Here's how the part is built. I have some questions about the finished solid (model axes, mm). Face numbers are marked on the shaded views. A direction names the side the tool comes from. Round coordinates to 2 decimals unless told otherwise and drop trailing zeros. Order: outer loops, then holes, each group sorted by start corner. A loop starts at its lowest first (then second) coordinate and runs counter-clockwise, first axis right, second up. Notation, with made-up numbers: (-21, -10) -> (14, -10) arc R14 ccw to (14, 3) -> close; hole circle Ø11 at (0, 31). An arc over 180 degrees is marked (long way). One line per item, written item: value.
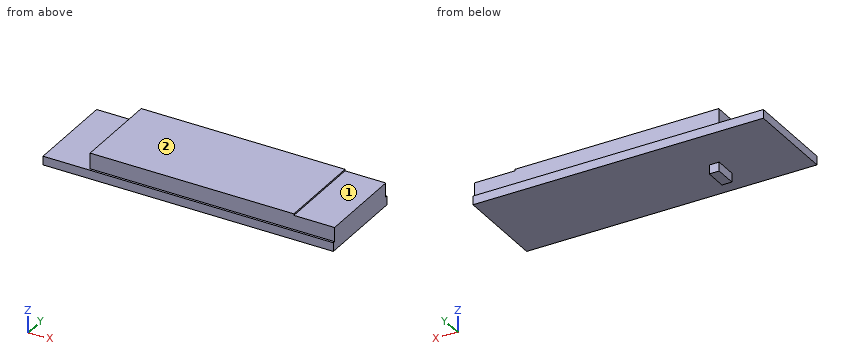
```python
from build123d import *

# Parameters (mm, degrees)
SKETCH_1_W      = 38
SKETCH_1_H      = 12
EXTRUDE_1_DEPTH = 1.14
SKETCH_2_W      = 1.3
SKETCH_2_H      = 2.84
EXTRUDE_2_DEPTH = 1.17
SKETCH_3_W      = 32
SKETCH_3_H      = 11.44
EXTRUDE_3_DEPTH = 1.86
SKETCH_4_W      = 26.67
SKETCH_4_H      = 11.44
EXTRUDE_4_DEPTH = 0.2


with BuildPart() as part:
    # Эскиз1 → Бобышка-Вытянуть1 (new body)
    with BuildSketch(Plane.XY):
        Rectangle(SKETCH_1_W, SKETCH_1_H)
    extrude(amount=EXTRUDE_1_DEPTH)

    # Эскиз2 → Бобышка-Вытянуть2 (add)
    with BuildSketch(Plane(origin=(0, 0, 0), x_dir=(-1, 0, 0), z_dir=(0, 0, -1))):
        with Locations((9.13, -1.3)):
            Rectangle(SKETCH_2_W, SKETCH_2_H)
    extrude(amount=EXTRUDE_2_DEPTH)

    # Эскиз3 → Бобышка-Вытянуть3 (add)
    with BuildSketch(Plane.XY.offset(1.14)):
        with Locations((3, 0)):
            Rectangle(SKETCH_3_W, SKETCH_3_H)
    extrude(amount=EXTRUDE_3_DEPTH)

    # Эскиз4 → Бобышка-Вытянуть4 (add)
    with BuildSketch(Plane.XY.offset(3)):
        with Locations((0.335, 0)):
            Rectangle(SKETCH_4_W, SKETCH_4_H)
    extrude(amount=EXTRUDE_4_DEPTH)


solid = part.part
```
Q1. I need wall thicknesses on line 1 along Z through (x, y) = (10, 2.25); line 2 along Y through (x, z) = (7.5, 1.25); line 3 along Z through (x, y) = (17.5, -1.5). Which ranges of each line are inside material? Lowest first, please.
Answers:
line 1: 0 to 3.2
line 2: -5.72 to 5.72
line 3: 0 to 3
Q2. I want a section at D-D on x = 15.5. Write out the boundary of the cut face in (y, z).
Answers:
outline: (-6, 0) -> (6, 0) -> (6, 1.14) -> (5.72, 1.14) -> (5.72, 3) -> (-5.72, 3) -> (-5.72, 1.14) -> (-6, 1.14) -> close
Q3. I want a section at B-B on y = -1.25. Write out the boundary of the cut face in (x, z), then the cut area to 3 significant figures.
Answers:
outline: (-19, 0) -> (-9.78, 0) -> (-9.78, -1.17) -> (-8.48, -1.17) -> (-8.48, 0) -> (19, 0) -> (19, 3) -> (13.67, 3) -> (13.67, 3.2) -> (-13, 3.2) -> (-13, 1.14) -> (-19, 1.14) -> close
area: 110 mm2
Q4. For P1, Ø1.6, axis at x = 4, z = 2.5, coming from the -Y side; P2, Ø6, axis at x = -5, y = -2.5, coming from the -Z side; P3, Ø6, axis at x = 17, y = 2.5, coming from the +Z side, each with a flat end and sliding along its axis, tell me the tip position at first contact or that it passes through.
Answers:
P1: y = -5.72
P2: z = 0
P3: z = 3
Q5. I want a section at C-C on z = 1.75. Write out the boundary of the cut face in (x, y), then the cut area to 3 significant figures.
Answers:
outline: (-13, -5.72) -> (19, -5.72) -> (19, 5.72) -> (-13, 5.72) -> close
area: 366 mm2
Q6. I want a section at A-A on x = 9. Write out the boundary of the cut face in (y, z), then the cut area to 3 significant figures.
Answers:
outline: (-6, 0) -> (6, 0) -> (6, 1.14) -> (5.72, 1.14) -> (5.72, 3.2) -> (-5.72, 3.2) -> (-5.72, 1.14) -> (-6, 1.14) -> close
area: 37.2 mm2
Q7. Which directions (+Z, -Z, +X, -X, +Y, -Y) give clear straight access to the entire face, cutting with the end or side of a thin tool? Please do the marked faces 1 and 2.
Answers:
face 1: +Z, +X, +Y, -Y
face 2: +Z, +X, -X, +Y, -Y
